Check sheet for the drawn part. Datum: minimum x, y, z corner. Units: mm. Round coordinates to 2 decimals unless told otherwise and drop trailing zeros. Loops run counter-clockwise (first coordinate to the right, second up) from the corner with the lowest first, then second, coordinate; pieces in that order, holes last. Notation, with made-up numbers: (-19, 42) - (-6, 42) arc R27 ccw to (-6, 60) - close; hole circle Ø10 at (71.5, -19). An arc over 180 degrees is marked (long way). Use CSV: the item, a comma, the result in double quotes.
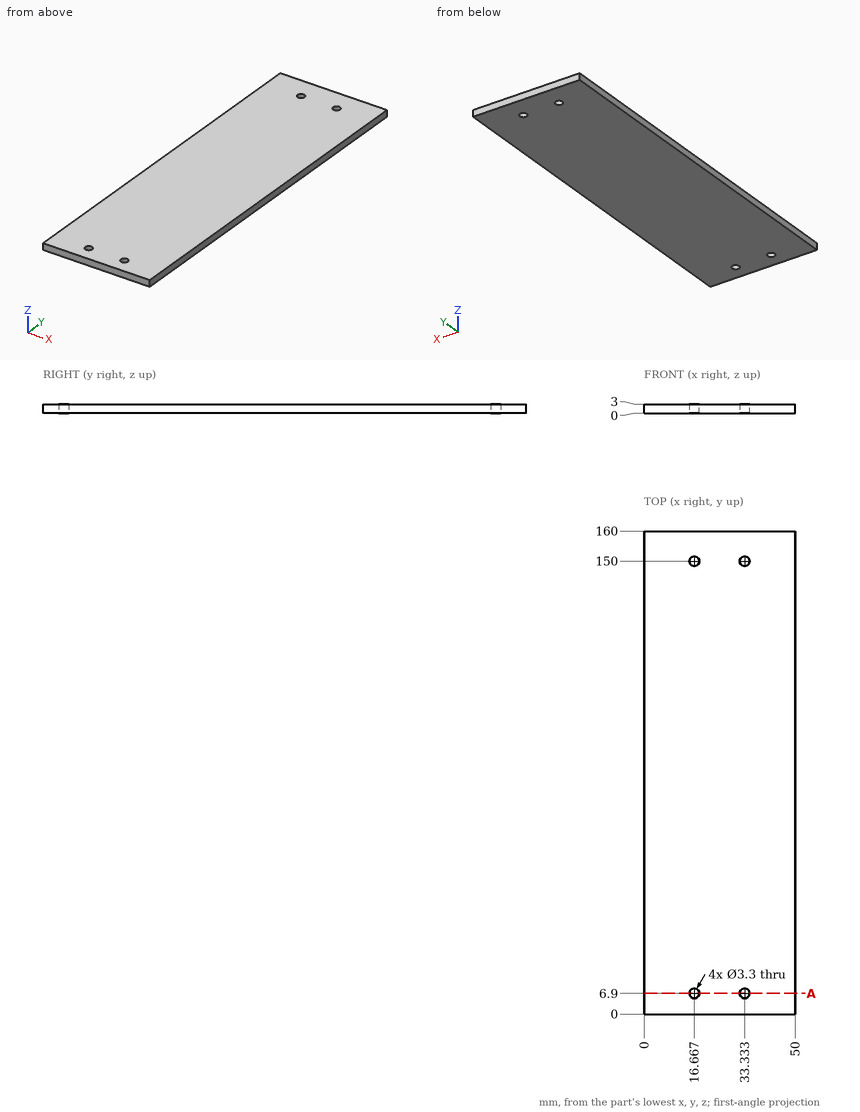
1) Cross-section at A-A, the plane y = 6.9. Record the cut outline in (x, z), then the cut area to 3 significant figures.
Returned:
outline,"(0, 0) - (15.02, 0) - (15.02, 3) - (0, 3) - close; (18.32, 0) - (31.68, 0) - (31.68, 3) - (18.32, 3) - close; (34.98, 0) - (50, 0) - (50, 3) - (34.98, 3) - close"
area,"130 mm²"
2) Gauge pin test, flat end, axial feed: pin 1 Ø1.5 at (x, y) = (12, 99.5) entering from -Z. Record the tip position at first contact, or that the pin passes through.
Returned:
pin 1,"stops at z = 0"
3) Thickness scan on probe 1 along X at (y, z) = (6.9, 1.4); probe 2 along Y at (x, z) = (18, 2.9); probe 3 along Y at (x, z) = (34, 1.65). Record the ranges inside material, lowest first. Write a range as [from, to].
Returned:
probe 1,"x = [0, 15.02], [18.32, 31.68], [34.98, 50]"
probe 2,"y = [0, 5.93], [7.87, 149.03], [150.97, 160]"
probe 3,"y = [0, 5.39], [8.41, 148.49], [151.51, 160]"
